from build123d import *

# Parameters (mm, degrees)
SKETCH1_R                                           = 1.65
SKETCH1_R_2                                         = 1.75
BOSS_EXTRUDE1_DEPTH                                 = 6
CSK_FOR_M3_COUNTERSUNK_FLAT_HEAD_SCREW1_D           = 3.6
CSK_FOR_M3_COUNTERSUNK_FLAT_HEAD_SCREW1_DEPTH       = 47
CSK_FOR_M3_COUNTERSUNK_FLAT_HEAD_SCREW1_CSINK_D     = 6.3
CSK_FOR_M3_COUNTERSUNK_FLAT_HEAD_SCREW1_CSINK_ANGLE = 90
CSK_FOR_M3_COUNTERSUNK_FLAT_HEAD_SCREW1_TIP         = 1.081549114
BOSS_EXTRUDE2_DEPTH                                 = 6
BOSS_EXTRUDE3_START                                 = 1.4
SKETCH5_R                                           = 6
SKETCH5_R_2                                         = 1.8
BOSS_EXTRUDE3_DEPTH                                 = 1.4
BOSS_EXTRUDE4_START                                 = 11
SKETCH6_R                                           = 4.975
SKETCH6_R_2                                         = 1.8
BOSS_EXTRUDE4_DEPTH                                 = 11
CHAMFER1_SIZE                                       = 1
CHAMFER1_SIZE2                                      = 0.5
CUT_EXTRUDE4_DEPTH                                  = 4.4
CHAMFER2_SIZE                                       = 0.5


with BuildPart() as part:
    # Sketch1 → Boss-Extrude1 (new body)
    with BuildSketch(Plane.XY):
        with BuildLine():
            Line((5, 7.483314774), (5, 25))
            ThreePointArc((5, 25), (3.828427125, 27.828427125), (1, 29))
            Line((1, 29), (-1, 29))
            ThreePointArc((-1, 29), (-3.828427125, 27.828427125), (-5, 25))
            Line((-5, 25), (-5, 7.483314774))
            ThreePointArc((-5, 7.483314774), (-9, 0), (-5, -7.483314774))
            Line((-5, -7.483314774), (-5, -15))
            ThreePointArc((-5, -15), (-3.828427125, -17.828427125), (-1, -19))
            Line((-1, -19), (1, -19))
            ThreePointArc((1, -19), (3.828427125, -17.828427125), (5, -15))
            Line((5, -15), (5, -7.483314774))
            ThreePointArc((5, -7.483314774), (9, 0), (5, 7.483314774))
        make_face()
        with Locations((0, 25)):
            Circle(SKETCH1_R, mode=Mode.SUBTRACT)
        with BuildLine():
            Line((-6.988562084, -0.4), (-3.979949748, -0.4))
            ThreePointArc((-3.979949748, -0.4), (-3.464101615, -2), (-2.336385036, -3.246737588))
            Line((-2.336385036, -3.246737588), (-3.840691203, -5.852272301))
            ThreePointArc((-3.840691203, -5.852272301), (-6.062177826, -3.5), (-6.988562084, -0.4))
        make_face(mode=Mode.SUBTRACT)
        with BuildLine():
            ThreePointArc((-1.643564713, -3.646737588), (0, -4), (1.643564713, -3.646737588))
            Line((1.643564713, -3.646737588), (3.14787088, -6.252272301))
            ThreePointArc((3.14787088, -6.252272301), (0, -7), (-3.14787088, -6.252272301))
            Line((-3.14787088, -6.252272301), (-1.643564713, -3.646737588))
        make_face(mode=Mode.SUBTRACT)
        with BuildLine():
            ThreePointArc((2.336385036, -3.246737588), (3.464101615, -2), (3.979949748, -0.4))
            Line((3.979949748, -0.4), (6.988562084, -0.4))
            ThreePointArc((6.988562084, -0.4), (6.062177826, -3.5), (3.840691203, -5.852272301))
            Line((3.840691203, -5.852272301), (2.336385036, -3.246737588))
        make_face(mode=Mode.SUBTRACT)
        with BuildLine():
            ThreePointArc((3.979949748, 0.4), (3.464101615, 2), (2.336385036, 3.246737588))
            Line((2.336385036, 3.246737588), (3.840691203, 5.852272301))
            ThreePointArc((3.840691203, 5.852272301), (6.062177826, 3.5), (6.988562084, 0.4))
            Line((6.988562084, 0.4), (3.979949748, 0.4))
        make_face(mode=Mode.SUBTRACT)
        with BuildLine():
            ThreePointArc((1.643564713, 3.646737588), (0, 4), (-1.643564713, 3.646737588))
            Line((-1.643564713, 3.646737588), (-3.14787088, 6.252272301))
            ThreePointArc((-3.14787088, 6.252272301), (0, 7), (3.14787088, 6.252272301))
            Line((3.14787088, 6.252272301), (1.643564713, 3.646737588))
        make_face(mode=Mode.SUBTRACT)
        with BuildLine():
            ThreePointArc((-2.336385036, 3.246737588), (-3.464101615, 2), (-3.979949748, 0.4))
            Line((-3.979949748, 0.4), (-6.988562084, 0.4))
            ThreePointArc((-6.988562084, 0.4), (-6.062177826, 3.5), (-3.840691203, 5.852272301))
            Line((-3.840691203, 5.852272301), (-2.336385036, 3.246737588))
        make_face(mode=Mode.SUBTRACT)
        with Locations((0, -15)):
            Circle(SKETCH1_R, mode=Mode.SUBTRACT)
        Circle(SKETCH1_R_2, mode=Mode.SUBTRACT)
    extrude(amount=BOSS_EXTRUDE1_DEPTH)

    # CSK for M3 Countersunk Flat Head Screw1
    with Locations(Plane.XY.offset(6)):
        with Locations((0, 0)):
            CounterSinkHole(CSK_FOR_M3_COUNTERSUNK_FLAT_HEAD_SCREW1_D / 2, CSK_FOR_M3_COUNTERSUNK_FLAT_HEAD_SCREW1_CSINK_D / 2, depth=CSK_FOR_M3_COUNTERSUNK_FLAT_HEAD_SCREW1_DEPTH, counter_sink_angle=CSK_FOR_M3_COUNTERSUNK_FLAT_HEAD_SCREW1_CSINK_ANGLE)
            with Locations((0, 0, -(CSK_FOR_M3_COUNTERSUNK_FLAT_HEAD_SCREW1_DEPTH + CSK_FOR_M3_COUNTERSUNK_FLAT_HEAD_SCREW1_TIP / 2))):  # 118° drill point
                Cone(0, CSK_FOR_M3_COUNTERSUNK_FLAT_HEAD_SCREW1_D / 2, CSK_FOR_M3_COUNTERSUNK_FLAT_HEAD_SCREW1_TIP, mode=Mode.SUBTRACT)

    # Sketch1<5> → Boss-Extrude2 (add)
    with BuildSketch(Plane.XY):
        with BuildLine():
            Line((3.640691203, 5.505862139), (2.336385036, 3.246737588))
            ThreePointArc((2.336385036, 3.246737588), (3.464101615, 2), (3.979949748, 0.4))
            Line((3.979949748, 0.4), (6.988562084, 0.4))
            ThreePointArc((6.988562084, 0.4), (6.062177826, 3.5), (3.840691203, 5.852272301))
            Line((3.840691203, 5.852272301), (3.640691203, 5.505862139))
        make_face()
        with BuildLine():
            Line((-2.94787088, 5.905862139), (-1.643564713, 3.646737588))
            ThreePointArc((-1.643564713, 3.646737588), (0, 4), (1.643564713, 3.646737588))
            Line((1.643564713, 3.646737588), (3.14787088, 6.252272301))
            ThreePointArc((3.14787088, 6.252272301), (0, 7), (-3.14787088, 6.252272301))
            Line((-3.14787088, 6.252272301), (-2.94787088, 5.905862139))
        make_face()
        with BuildLine():
            ThreePointArc((-2.336385036, -3.246737588), (-3.464101615, -2), (-3.979949748, -0.4))
            Line((-3.979949748, -0.4), (-6.988562084, -0.4))
            ThreePointArc((-6.988562084, -0.4), (-6.062177826, -3.5), (-3.840691203, -5.852272301))
            Line((-3.840691203, -5.852272301), (-3.640691203, -5.505862139))
            Line((-3.640691203, -5.505862139), (-2.336385036, -3.246737588))
        make_face()
        with BuildLine():
            Line((-6.588562084, 0.4), (-3.979949748, 0.4))
            ThreePointArc((-3.979949748, 0.4), (-3.464101615, 2), (-2.336385036, 3.246737588))
            Line((-2.336385036, 3.246737588), (-3.840691203, 5.852272301))
            ThreePointArc((-3.840691203, 5.852272301), (-6.062177826, 3.5), (-6.988562084, 0.4))
            Line((-6.988562084, 0.4), (-6.588562084, 0.4))
        make_face()
        with BuildLine():
            ThreePointArc((3.979949748, -0.4), (3.464101615, -2), (2.336385036, -3.246737588))
            Line((2.336385036, -3.246737588), (3.840691203, -5.852272301))
            ThreePointArc((3.840691203, -5.852272301), (6.062177826, -3.5), (6.988562084, -0.4))
            Line((6.988562084, -0.4), (6.588562084, -0.4))
            Line((6.588562084, -0.4), (3.979949748, -0.4))
        make_face()
        with BuildLine():
            ThreePointArc((1.643564713, -3.646737588), (0, -4), (-1.643564713, -3.646737588))
            Line((-1.643564713, -3.646737588), (-3.14787088, -6.252272301))
            ThreePointArc((-3.14787088, -6.252272301), (0, -7), (3.14787088, -6.252272301))
            Line((3.14787088, -6.252272301), (2.94787088, -5.905862139))
            Line((2.94787088, -5.905862139), (1.643564713, -3.646737588))
        make_face()
    extrude(amount=BOSS_EXTRUDE2_DEPTH)

    # Sketch5 → Boss-Extrude3 (add)
    with BuildSketch(Plane(origin=(0, 0, 0), x_dir=(-1, 0, 0), z_dir=(0, 0, -1)).offset(BOSS_EXTRUDE3_START)):
        Circle(SKETCH5_R)
        with Locations(Location((0, 0, 0), (0, 0, 180))):
            Circle(SKETCH5_R_2, mode=Mode.SUBTRACT)
    extrude(amount=-BOSS_EXTRUDE3_DEPTH)

    # Sketch6 → Boss-Extrude4 (add)
    with BuildSketch(Plane(origin=(0, 0, -1.4), x_dir=(-1, 0, 0), z_dir=(0, 0, -1)).offset(BOSS_EXTRUDE4_START)):
        Circle(SKETCH6_R)
        with Locations(Location((0, 0, 0), (0, 0, 180))):
            Circle(SKETCH6_R_2, mode=Mode.SUBTRACT)
    extrude(amount=-BOSS_EXTRUDE4_DEPTH)

    # Chamfer1
    chamfer1_edges = [part.edges().sort_by_distance(p)[0] for p in [
        (4.975, 0, -12.4),
    ]]
    chamfer1_side = [part.faces().sort_by_distance(p)[0] for p in [
        (4.975, 0, -6.9),
    ]]
    chamfer(chamfer1_edges, length=CHAMFER1_SIZE, length2=CHAMFER1_SIZE2, reference=chamfer1_side[0])

    # Sketch7 → Cut-Extrude4 (cut)
    with BuildSketch(Plane(origin=(0, 0, 0), x_dir=(-1, 0, 0), z_dir=(0, 0, -1))):
        Polygon((2.85, 23.354551733), (2.85, 26.645448267), (0, 28.290896534), (-2.85, 26.645448267), (-2.85, 23.354551733), (0, 21.709103466), align=None)
        Polygon((2.85, -13.354551733), (0, -11.709103466), (-2.85, -13.354551733), (-2.85, -16.645448267), (0, -18.290896534), (2.85, -16.645448267), align=None)
    extrude(amount=-CUT_EXTRUDE4_DEPTH, mode=Mode.SUBTRACT)

    # Chamfer2
    chamfer2_edges = [part.edges().sort_by_distance(p)[0] for p in [
        (-5, -11.241657387, 6),
        (-3.828427125, -17.828427125, 6),
        (0, -19, 6),
        (3.828427125, -17.828427125, 6),
        (5, -11.241657387, 6),
        (9, 0, 6),
        (5, 16.241657387, 6),
        (3.828427125, 27.828427125, 6),
        (0, 29, 6),
        (-3.828427125, 27.828427125, 6),
        (-5, 16.241657387, 6),
        (-9, 0, 6),
    ]]
    chamfer(chamfer2_edges, length=CHAMFER2_SIZE)


solid = part.part
Work out the finished part from the listing and answer in its coordinate system (mm). A direction names the side the tool comes from. Round coordinates to 2 decimals unless told otherwise and drop trailing zeros. Write each loop counter-clockwise with the first axis right and the second up, starting at its lowest first coordinate (ties: lowest second). Pieces come first, ordered by that corner, then holes.
1) Straight lines are drawn through the part: line 1 (Y direction, x = 0, z = 4.5); line 2 (Y direction, x = 0, z = 4.8); line 3 (X direction, y = -15, z = 5.1). For each, find the intervals that lie inside material, in ascending order.
2) A tool of negligible diameter and unlimited length cuts with its end or side. For faces 1 (the flat face through (5, -11, 3)), 2 (the conical face through (-3.599, -17.542, 5.865)), 3 (the flat face through (-1.44, -12.54, 2.17)), from which of +Z, -Z, +X, -X, +Y, -Y can it reach the whole face along a straight path? Write none if from no direction.
3) A cutting plane is placed at B-B (y = 0). Give the vertices of the cut face in (x, z) (3 decimals).
4) The mould has two halves that part along Y. Classify faces 4 (the flat face through (-1.405, -17.48, 2.169)), 5 (the conical face through (3.599, 27.542, 5.865)), 6 (the flat face through (1.44, 22.54, 2.17)), 7 (the cylindrical face through (9, 0, 3)): pulls with the +Y half, pulls with the -Y half, needs draft (parallel to the pull), parting line crosses it, or undercut.
5) A cutting plane is placed at C-C (y = 15.5). Give the vertices of the cut face in (x, z), plus the area to 4 significant figures.
6) A cutting plane is placed at D-D (z = -10.5). Give the vertices of the cut face in (x, y) (3 decimals).
7) Given pin 1 Ø3 at (y, z) = (17, 2.5) entering from +X; pin 2 Ø8 at (x, z) = (-5.5, -5) entering from +Y; pin 3 Ø3 at (y, z) = (20, 4) entering from -X; pin 4 Ø3 at (x, y) = (0, 0) entering from -Z, each flat-ended and moving along its own axis, determine where each tip first touches the part or whether it passes through.
8) A cutting plane is placed at A-A (z = 2.5). Give the vertices of the cut face in (x, y).
Completed:
1. line 1: y = -19 to -16.65, -13.35 to -1.8, 1.8 to 23.35, 26.65 to 29
1. line 2: y = -19 to -16.65, -13.35 to -1.95, 1.95 to 23.35, 26.65 to 29
1. line 3: x = -5 to -1.65, 1.65 to 5
2. face 1: +Z, -Z, +X, -Y
2. face 2: +Z, -X, -Y
2. face 3: -Z
3. outline: (-9, 0) - (-6, 0) - (-6, -1.4) - (-4.975, -1.4) - (-4.975, -11.4) - (-4.475, -12.4) - (-1.8, -12.4) - (-1.8, 4.65) - (-3.15, 6) - (-8.5, 6) - (-9, 5.5) - close; (1.8, -12.4) - (4.475, -12.4) - (4.975, -11.4) - (4.975, -1.4) - (6, -1.4) - (6, 0) - (9, 0) - (9, 5.5) - (8.5, 6) - (3.15, 6) - (1.8, 4.65) - close
4. face 4: undercut
4. face 5: pulls with the +Y half
4. face 6: undercut
4. face 7: parting line crosses it
5. outline: (-5, 0) - (5, 0) - (5, 5.5) - (4.5, 6) - (-4.5, 6) - (-5, 5.5) - close
5. area: 59.75 mm2
6. outline: circle Ø9.95 at (0, 0); hole circle Ø3.6 at (0, 0)
7. pin 1: stops at x = 5
7. pin 2: stops at y = 4.74
7. pin 3: stops at x = -5
7. pin 4: passes through
8. outline: (-5, -15) arc R4 ccw to (-1, -19) - (1, -19) arc R4 ccw to (5, -15) - (5, -7.48) arc R9 ccw to (5, 7.48) - (5, 25) arc R4 ccw to (1, 29) - (-1, 29) arc R4 ccw to (-5, 25) - (-5, 7.48) arc R9 ccw to (-5, -7.48) - close; hole (-2.85, -16.65) - (0, -18.29) - (2.85, -16.65) - (2.85, -13.35) - (0, -11.71) - (-2.85, -13.35) - close; hole (-2.85, 23.35) - (0, 21.71) - (2.85, 23.35) - (2.85, 26.65) - (0, 28.29) - (-2.85, 26.65) - close; hole circle Ø3.6 at (0, 0)
